from build123d import *

# Parameters (mm, degrees)
BOX032_W              = 10
BOX032_H              = 10
BOX032_DEPTH          = 30
CYLINDER003_R         = 1.7
CYLINDER003_DEPTH     = 30
BOX022_W              = 1.5
BOX022_H              = 7.8
BOX022_DEPTH          = 8
CHAMFER006006003_SIZE = 1.49
BOX020_W              = 1.5
BOX020_H              = 7.8
BOX020_DEPTH          = 12
CHAMFER_SIZE          = 1.49
BOX021_W              = 5
BOX021_H              = 7.8
BOX021_DEPTH          = 5
BOX_W                 = 2
BOX_H                 = 2
BOX_DEPTH             = 30
CHAMFER006006002_SIZE = 1
CYLINDER002_R         = 5
CYLINDER002_DEPTH     = 30
CYLINDER001_R         = 11
CYLINDER001_DEPTH     = 10
CYLINDER_R            = 4
CYLINDER_DEPTH        = 10
BOX019_W              = 6
BOX019_H              = 30
BOX019_DEPTH          = 30
CHAMFER006006004_SIZE = 2
CHAMFER006006005_SIZE = 0.99
CHAMFER006006019_SIZE = 0.4


with BuildPart() as cube031:
    # Box032 → Box032 (new body)
    with BuildSketch(Plane(origin=(-3.5, 22, 0), x_dir=(1, 0, 0), z_dir=(0, 0, 1))):
        with Locations((5, 5)):
            Rectangle(BOX032_W, BOX032_H)
    extrude(amount=BOX032_DEPTH)


with BuildPart() as cylinder003:
    # Cylinder003 → Cylinder003 (new body)
    with BuildSketch(Plane(origin=(-6, -1, 0), x_dir=(1, 0, 0), z_dir=(0, 0, 1))):
        Circle(CYLINDER003_R)
    extrude(amount=CYLINDER003_DEPTH)


with BuildPart() as chamfer006006003:
    # Box022 → Box022 (new body)
    with BuildSketch(Plane(origin=(0, 11.1, 22), x_dir=(1, 0, 0), z_dir=(0, 0, 1))):
        with Locations((0.75, 3.9)):
            Rectangle(BOX022_W, BOX022_H)
    extrude(amount=BOX022_DEPTH)

    # Chamfer006006003
    chamfer006006003_edges = [chamfer006006003.edges().sort_by_distance(p)[0] for p in [
        (1.5, 15, 22),
    ]]
    chamfer(chamfer006006003_edges, length=CHAMFER006006003_SIZE)


with BuildPart() as chamfer_body:
    # Box020 → Box020 (new body)
    with BuildSketch(Plane(origin=(0, 11.1, 0), x_dir=(1, 0, 0), z_dir=(0, 0, 1))):
        with Locations((0.75, 3.9)):
            Rectangle(BOX020_W, BOX020_H)
    extrude(amount=BOX020_DEPTH)

    # Chamfer
    chamfer_edges = [chamfer_body.edges().sort_by_distance(p)[0] for p in [
        (1.5, 15, 12),
    ]]
    chamfer(chamfer_edges, length=CHAMFER_SIZE)


with BuildPart() as cube020:
    # Box021 → Box021 (new body)
    with BuildSketch(Plane(origin=(0, 11.1, 0), x_dir=(1, 0, 0), z_dir=(0, 0, 1))):
        with Locations((2.5, 3.9)):
            Rectangle(BOX021_W, BOX021_H)
    extrude(amount=BOX021_DEPTH)


with BuildPart() as chamfer006006002:
    # Box → Box (new body)
    with BuildSketch(Plane(origin=(-2, -1, 0), x_dir=(1, 0, 0), z_dir=(0, 0, 1))):
        with Locations((1, 1)):
            Rectangle(BOX_W, BOX_H)
    extrude(amount=BOX_DEPTH)

    # Chamfer006006002
    chamfer006006002_edges = [chamfer006006002.edges().sort_by_distance(p)[0] for p in [
        (0, -1, 15),
    ]]
    chamfer(chamfer006006002_edges, length=CHAMFER006006002_SIZE)


with BuildPart() as cylinder002:
    # Cylinder002 → Cylinder002 (new body)
    with BuildSketch(Plane(origin=(-6, -1, 0), x_dir=(1, 0, 0), z_dir=(0, 0, 1))):
        Circle(CYLINDER002_R)
    extrude(amount=CYLINDER002_DEPTH)


with BuildPart() as cylinder001:
    # Cylinder001 → Cylinder001 (new body)
    with BuildSketch(Plane(origin=(-5, 15, 17), x_dir=(0, 0, 1), z_dir=(-1, 0, 0))):
        Circle(CYLINDER001_R)
    extrude(amount=CYLINDER001_DEPTH)


with BuildPart() as cylinder:
    # Cylinder → Cylinder (new body)
    with BuildSketch(Plane(origin=(3, 15, 17), x_dir=(0, 0, 1), z_dir=(-1, 0, 0))):
        Circle(CYLINDER_R)
    extrude(amount=CYLINDER_DEPTH)


with BuildPart() as chamfer006006019:
    # Box019 → Box019 (new body)
    with BuildSketch(Plane(origin=(-6, 0, 0), x_dir=(1, 0, 0), z_dir=(0, 0, 1))):
        with Locations((3, 15)):
            Rectangle(BOX019_W, BOX019_H)
    extrude(amount=BOX019_DEPTH)

    # Chamfer006006004
    chamfer006006004_edges = [chamfer006006019.edges().sort_by_distance(p)[0] for p in [
        (-3, 30, 0),
        (-3, 30, 30),
    ]]
    chamfer(chamfer006006004_edges, length=CHAMFER006006004_SIZE)

    # Cut: cut Cylinder
    add(cylinder.part, mode=Mode.SUBTRACT)

    # Cut001: cut Cylinder001
    add(cylinder001.part, mode=Mode.SUBTRACT)

    # Chamfer006006005
    chamfer006006005_edges = [chamfer006006019.edges().sort_by_distance(p)[0] for p in [
        (-5, 15, 6),
    ]]
    chamfer(chamfer006006005_edges, length=CHAMFER006006005_SIZE)

    # Fusion: union Chamfer006006003, Chamfer body, Cube020, Chamfer006006002, Cylinder002
    add(chamfer006006003.part)
    add(chamfer_body.part)
    add(cube020.part)
    add(chamfer006006002.part)
    add(cylinder002.part)

    # Cut002: cut Cylinder003
    add(cylinder003.part, mode=Mode.SUBTRACT)

    # Cut002004005003: cut Cube031
    add(cube031.part, mode=Mode.SUBTRACT)

    # Chamfer006006019
    chamfer006006019_edges = [chamfer006006019.edges().sort_by_distance(p)[0] for p in [
        (-0.5, -0.5, 0),
        (-0.5, -0.5, 30),
        (0, 20.45, 0),
        (-1.75, 22, 0),
        (-3.5, 25, 0),
        (-6, 16, 0),
        (-9.535534, -4.535534, 0),
        (0, 5.55, 0),
        (2.5, 11.1, 0),
        (5, 15, 0),
        (2.5, 18.9, 0),
        (-7.202082, -2.202082, 0),
        (-5.228638, 0.514926, 0),
        (-4.38335, -0.474221, 0),
        (0, 5.55, 30),
        (0, 20.45, 30),
        (-6, 16, 30),
        (-3.5, 25, 30),
        (-1.75, 22, 30),
        (0.75, 18.9, 30),
        (1.5, 15, 30),
        (0.75, 11.1, 30),
        (-9.535534, -4.535534, 30),
        (-7.202082, -2.202082, 30),
        (-5.228638, 0.514926, 30),
        (-4.38335, -0.474221, 30),
        (-3.5, 29, 29),
        (-3.5, 30, 15),
        (-3.5, 29, 1),
        (-6, 29, 1),
        (-6, 29, 29),
        (-6, 30, 15),
    ]]
    chamfer(chamfer006006019_edges, length=CHAMFER006006019_SIZE)


with BuildPart() as chamfer006006019_1:
    # Chamfer006006019 placement: moved
    add(chamfer006006019.part.moved(Location((0, 0, 5))))


solid = chamfer006006019_1.part
Geometry check sheet. Reference: the model listing, model coordinates, mm. A direction names the side the tool comes from. Give positions to 0.01 mm unless a question says otherwise; leave off trailing zeros. Loops run counter-clockwise (first coordinate to the right, second up) from the corner with the lowest first, then second, coordinate; pieces in that order, holes last. Notation, with made-up numbers: M 10,75.5 L 32,75.5 A22 cw 32,114.5 Z; hole C 76.25,67 d4. An arc over 180 degrees is marked long. Write each question's results on one line, items separated by ' | '.
1) Release check for a two-part mould opening along Z. For faces 4 (the face through (0.74, 14.95, 16.27)), 5 (the face through (-5, 29, 6)), 6 (the face through (-6, 22, 13)) record: +Z half, -Z half, draft (parallel to the pull), parting line (faces both ways), or undercut.
Answers follow:
face 4: undercut | face 5: -Z half | face 6: draft
2) Tool access check on faces 1 (the face through (-0.71, -0.43, 5.2)), 2 (the face through (-5, 10.7, 21.9)), 3 (the face through (0.74, 14.95, 27.73)). Record the directions out of +Z, -Z, +X, -X, +Y, -Y that give a thin tool (end or side, any length) a straight path to the whole face; none if there is none.
Answers follow:
face 1: -Z, +X, -Y | face 2: -X | face 3: +X, +Y, -Y
3) Gauge pin test, flat ends, axial feed: pin 1 (8 mm diameter, centred on y = 20, z = 22.5, fed in from +X); pin 2 (6 mm diameter, centred on y = 26, z = 22.5, fed in from +X); pin 3 (3 mm diameter, centred on y = 16.5, z = 30.5, fed in from +X); pin 4 (12 mm diameter, centred on y = 2.5, z = 15.5, fed in from -X). Record the tip position at first contact, or that the pin passes through.
Answers follow:
pin 1: x = 0 | pin 2: x = -3.5 | pin 3: x = 1.5 | pin 4: x = -11
4) Section check B-B, the plane x = 3.25. Record the boundary of the cut face in (y, z), plus the area to 3 significant figures.
Answers follow:
outline: M 11.1,5.4 L 11.5,5 L 18.5,5 L 18.9,5.4 L 18.9,10 L 11.1,10 Z | area: 38.8 mm2
5) Thickness scan on line 1 (Z direction, x = -2.5, y = 15); line 2 (X direction, y = 28, z = 8); line 3 (Y direction, x = -3.6, z = 22). Record the ranges inside material, lowest first.
Answers follow:
line 1: 5 to 18, 26 to 35 | line 2: -6 to -3.5 | line 3: -5.39 to 11, 19 to 29.7
6) Section check C-C, the plane z = 24. Count the separate pieces of the cut face and the enclosed holes in it, plus the area to 3 significant figures.
Answers follow:
separate pieces: 2 | enclosed holes: 1 | area: 152 mm2
